Read the model definition and answer for the solid it produces. Units are mm, in the model's axes. A direction names the side the tool comes from. Round coordinates to 2 decimals unless told otherwise and drop trailing zeros. Write each loop counter-clockwise with the first axis right and the second up, starting at its lowest first coordinate (ties: lowest second). Pieces come first, ordered by that corner, then holes. Notation, with made-up numbers: (37.25, 88) - (72.25, 88) arc R18 cw to (72.25, 97) - close; hole circle Ø7 at (-19, -13.5). An arc over 180 degrees is marked (long way). Use one line per item in the form item = value. Start each with the question number.
1) Each of these flat-tipped pins is pushed along its axis until it touches: pin 1 (8 mm diameter, centred on x = -25.5, z = 6, fed in from +Y); pin 2 (2 mm diameter, centred on y = -48.5, z = 8.5, fed in from +X); pin 3 (5 mm diameter, centred on x = -14, z = 6.5, fed in from -Y); pin 4 (2 mm diameter, centred on x = -37, y = 42.5, fed in from -Z). Where does it stop, or does it pass through?
2) Consider line 1 along Y through (x, z) = (-28, 3.5); line 2 along Y through (x, z) = (-17, 1.5); line 3 along Y through (x, z) = (-34, 5.25). Determine where each line is inside the solid, lowest interval first. Write a range as from..to.
3) For faces 5 (the face through (-17, -25, 10)), 6 (the face through (-37, 21, 8)), 7 (the face through (-17, -19.626, 5)), 8 (the face through (-25, -74.865, 5)), determine the directions among +Z, -Z, +X, -X, +Y, -Y from which every point of the face is accessible in a straight line to the end or side of a thin tool.
4) The part is cut by section C-C, the plane x = -37. Give the vertices of the cut face in (y, z), plus the area to 3 significant figures.
5) For a pull along X with two mould halves and no side action, classify faces 1 (the face through (-41.925, 77.769, 4.085)), 2 (the face through (-26, 57.311, 5)), 3 (the face through (-25, 68.358, 5)), 4 (the face through (-37, 21, 4)) as released by +X, released by -X, zero draft, split by the parting line, or undercut.
6) The part is cut by section A-A, the plane x = -26.5. Count the separate pieces of the cut face and the enclosed holes in it, plus the area to 3 significant figures.
7) The part is cut by section B-B, the plane y = 23. Give the vertices of the cut face in (x, z).
8) The part is cut by section D-D, the plane y = -12. Give the vertices of the cut face in (x, z), plus the area to 3 significant figures.
from build123d import *

# Parameters (mm, degrees)
F1_DEPTH = 15
F0_W     = 25
F0_H     = 10
F0_W_2   = 2.5
F0_H_2   = 9.0467076302
F2_DEPTH = 10
F3_W     = 4
F3_H     = 4
F4_DEPTH = 100
F6_W     = 1
F6_H     = 1
F5_W     = 1
F5_H     = 1
F7_DEPTH = 30
F8_R     = 5
F8_R_2   = 4
F9_DEPTH = 15


with BuildPart() as f1:
    # F0 (on Top) → F1 (new body)
    with BuildSketch(Plane.XY):
        Polygon((-29.806669808, 70.373563841), (-44.806669808, 70.373563841), (-44.806669808, -79.626436159), (-29.806669808, -79.626436159), (-29.806669808, -74.8653486371), (-29.806669808, -72.8653486371), (-29.806669808, -63.8186410069), (-29.806669808, -61.8186410069), (-29.806669808, -29.626436159), (-29.806669808, -19.626436159), (-29.806669808, 20.373563841), (-29.806669808, 30.373563841), (-29.806669808, 55.3112663329), (-29.806669808, 57.3112663329), (-29.806669808, 66.357973963), (-29.806669808, 68.357973963), align=None)
    extrude(amount=F1_DEPTH)

    # F0 (on Top) → F2 (join)
    with BuildSketch(Plane.XY):
        with Locations((-17.306669808, 25.373563841)):
            Rectangle(F0_W, F0_H)
        with Locations((-17.306669808, -24.626436159)):
            Rectangle(F0_W, F0_H)
        Polygon((-29.806669808, -61.8186410069), (-29.806669808, -63.8186410069), (-22.306669808, -63.8186410069), (-19.806669808, -63.8186410069), (-19.806669808, -61.8186410069), align=None)
        with Locations((-21.056669808, -68.341994822)):
            Rectangle(F0_W_2, F0_H_2)
        Polygon((-29.806669808, -72.8653486371), (-29.806669808, -74.8653486371), (-19.806669808, -74.8653486371), (-19.806669808, -72.8653486371), (-22.306669808, -72.8653486371), align=None)
        Polygon((-22.3066698015, 57.3112663329), (-29.8066698015, 57.3112663329), (-29.806669808, 55.3112663329), (-19.8066698015, 55.3112663329), (-19.8066698015, 57.3112663329), align=None)
        with Locations((-21.0566698015, 61.8346201479)):
            Rectangle(F0_W_2, F0_H_2)
        Polygon((-19.8066698015, 68.357973963), (-29.8066698015, 68.357973963), (-29.806669808, 66.357973963), (-22.3066698015, 66.357973963), (-19.8066698015, 66.357973963), align=None)
    extrude(amount=F2_DEPTH)

    # F3 (on face) → F4 (cut)
    with BuildSketch(Plane(origin=(0, 70.373563841, 0), x_dir=(-1, 0, 0), z_dir=(0, 1, 0))):
        with Locations((36.806669808, 6)):
            Rectangle(F3_W, F3_H)
    extrude(amount=-F4_DEPTH, mode=Mode.SUBTRACT)

    # F6 (on face) + F5 (on face) → F7 (cut)
    with BuildSketch(Plane.YZ.offset(-4.806669808)):
        with Locations((25.373563841, 5)):
            Rectangle(F6_W, F6_H)
    with BuildSketch(Plane.YZ.offset(-4.806669808)):
        with Locations((-24.626436159, 5)):
            Rectangle(F5_W, F5_H)
    extrude(amount=-F7_DEPTH, mode=Mode.SUBTRACT)

    # F8 (on face) → F9 (join)
    with BuildSketch(Plane(origin=(0, 70.373563841, 0), x_dir=(-1, 0, 0), z_dir=(0, 1, 0))):
        with Locations((37.306669808, 6)):
            Circle(F8_R)
        with Locations((37.306669808, 6)):
            Circle(F8_R_2, mode=Mode.SUBTRACT)
    extrude(amount=F9_DEPTH)


solid = f1.part
Geometry results:
q1.pin_1 = 68.36
q1.pin_2 = -29.81
q1.pin_3 = -29.63
q1.pin_4 = 0
q2.line_1 = -74.87..-72.87, -63.82..-61.82, -29.63..-19.63, 20.37..30.37, 55.31..57.31, 66.36..68.36
q2.line_2 = -29.63..-19.63, 20.37..30.37
q2.line_3 = -79.63..-25.13, -24.13..24.87, 25.87..70.37
q3.face_5 = +Z, +X, +Y, -Y
q3.face_6 = +Y
q3.face_7 = +Z, -Z, +X
q3.face_8 = +Z, -Z, +X, -Y
q4.outline = (-79.63, 0) - (70.37, 0) - (70.37, 1.01) - (85.37, 1.01) - (85.37, 2.01) - (70.37, 2.01) - (70.37, 4) - (-29.63, 4) - (-29.63, 8) - (70.37, 8) - (70.37, 9.99) - (85.37, 9.99) - (85.37, 10.99) - (70.37, 10.99) - (70.37, 15) - (-79.63, 15) - close
q4.area = 1,880 mm2
q5.face_1 = split by the parting line
q5.face_2 = undercut
q5.face_3 = zero draft
q5.face_4 = undercut
q6.separate_pieces = 6
q6.enclosed_holes = 2
q6.area = 278 mm2
q7.outline = (-44.81, 0) - (-4.81, 0) - (-4.81, 10) - (-29.81, 10) - (-29.81, 15) - (-44.81, 15) - close; hole (-38.81, 4) - (-34.81, 4) - (-34.81, 8) - (-38.81, 8) - close
q8.outline = (-44.81, 0) - (-29.81, 0) - (-29.81, 15) - (-44.81, 15) - close; hole (-38.81, 4) - (-34.81, 4) - (-34.81, 8) - (-38.81, 8) - close
q8.area = 209 mm2
